The listing builds one solid part. Answer for the finished solid, in the listing's coordinates (mm). A direction names the side the tool comes from. Round coordinates to 2 decimals unless told otherwise and drop trailing zeros. Write each loop counter-clockwise with the first axis right and the second up, starting at its lowest first coordinate (ties: lowest second). Pieces come first, ordered by that corner, then holes. Notation, with made-up numbers: (39, -26) - (43, -26) arc R32 ccw to (43, 0) - close; hole circle Ø5 at (16, 10). An arc over 180 degrees is marked (long way). Return JSON: item names as keys, results as strings. Group by question number.
(1) Section C-C, the plane x = 261.5 is taken. Write down the section's boundary in (y, z), then the cut area to 3 significant figures.
(2) Determine the mould class of faces 1 (the flat face through (131, 21, 99)), 2 (the flat face through (0, 20, 50)) for opening direction X: +X half, -X half, draft (parallel to the pull), parting line (faces both ways), or undercut.
(3) Section B-B, the plane z = 53 is taken. Write down the section's boundary in (x, y).
(4) Which of the six approach directions +Z, -Z, +X, -X, +Y, -Y give full straight-line access (tool end or side, diameter ignored) to faces 3 (the flat face through (131, 40.8, 54)), 4 (the flat face through (271, 15, 94.5)), 5 (the flat face through (131, 20, 0))?
(5) Find the intervals of material crossed by line 1 along X through (y, z) = (30, 1); line 2 along Z through (x, y) = (148, 9); line 3 along Y through (x, z) = (158.5, 55), in increasing order. Write a range as [from, to].
(6) Section A-A, the plane y = 13 is taken. Write down the section's boundary in (x, z).
(7) Each of these flat-tipped pins is pushed along its axis until it touches: pin 1 (12 mm diameter, centred on x = 224, y = 20, fed in from -Z); pin 2 (0.5 mm diameter, centred on x = 265.5, z = -21, fed in from -Y); pin 3 (6 mm diameter, centred on y = 9, z = -5.5, fed in from +X). Where does it stop, or does it pass through?
Autodesk Inventor part; units mm, degrees
ref_plane "YZ Plane" through (0, 0, 0) normal (1, 0, 0) x (0, 1, 0)
ref_plane "XZ Plane" through (0, 0, 0) normal (0, 1, 0) x (-1, 0, 0)
ref_plane "XY Plane" through (0, 0, 0) normal (0, 0, 1) x (1, 0, 0)
sketch "Sketch1" plane through (0, 0, 0) normal (1, 0, 0) x (0, 1, 0)
  line L0 (0, 0) -> (40.8, 0)
  line L1 (40.8, 0) -> (40.8, 99)
  line L2 (40.8, 99) -> (0, 99)
  line L3 (0, 99) -> (0, 0)
  dimension "d0" = 40.8
  dimension "d1" = 99
extrude "Extrusion1" add sketch "Sketch1" along normal blind 265
sketch "Sketch2" plane through (265, 0, 0) normal (1, 0, 0) x (0, 0, -1)
  line L0 (0, 40.8) -> (-99, 40.8)
  line L1 (-94.5, 40.8) -> (-94.5, -1.5)
  line L2 (-94.5, -1.5) -> (-93.5, -1.5)
  line L3 (-93.5, -1.5) -> (-93.5, 1.8)
  line L4 (-93.5, 1.8) -> (14.5, 1.8)
  line L5 (14.5, 1.8) -> (18.5, 5.8)
  line L6 (18.5, 5.8) -> (26, 5.8)
  line L7 (26, 5.8) -> (26, 16.3)
  line L8 (26, 16.3) -> (18.5, 16.3)
  line L9 (18.5, 16.3) -> (14.5, 21.3)
  line L10 (14.5, 21.3) -> (18.5, 26.3)
  line L11 (18.5, 26.3) -> (26, 26.3)
  line L12 (26, 26.3) -> (26, 36.8)
  line L13 (26, 36.8) -> (18.5, 36.8)
  line L14 (18.5, 36.8) -> (14.5, 40.8)
  line L15 (14.5, 40.8) -> (0, 40.8)
  line L16 (0, 0) -> (0, 40.8)
  line L17 (0, 40.8) -> (-94.5, 40.8)
  line L18 (-99, 40.8) -> (-99, 0)
  line L19 (-99, 0) -> (0, 0)
  line L20 (14.5, 21.3) -> (14.5, 40.8) construction
  dimension "d4" = 4.5
  dimension "d5" = 1
  dimension "d6" = 1.5
  dimension "d7" = 135
  dimension "d8" = 135
  dimension "d9" = 10.5
  dimension "d10" = 4
  dimension "d11" = 7.5
  dimension "d13" = 10
  dimension "d14" = 108
extrude "Extrusion2" add sketch "Sketch2" along normal blind 1 contours L16 L4 L3 L19 L1 L0 | L15 L14 L13 L12 L11 L10 L9 L8 L7 L6 L5 L4 L16 | L19 L3 L2 L1
sketch "Sketch3" plane through (265, -1.5, 94.5) normal (0, 0, 1) x (1, 0, 0)
  line L0 (1, 42.3) -> (1, 0)
  line L1 (1, 0) -> (12.5, 0)
  line L2 (12.5, 0) -> (12.5, 8.05)
  line L3 (12.5, 8.05) -> (9.5, 8.05)
  line L4 (9.5, 8.05) -> (9.5, 11.05)
  line L5 (9.5, 11.05) -> (12.5, 11.05)
  line L6 (12.5, 11.05) -> (12.5, 28.55)
  line L7 (12.5, 28.55) -> (9.5, 28.55)
  line L8 (9.5, 28.55) -> (9.5, 31.55)
  line L9 (9.5, 31.55) -> (12.5, 31.55)
  line L10 (12.5, 31.55) -> (12.5, 39.7)
  line L11 (12.5, 39.7) -> (1, 39.7)
  line L12 (1, 39.7) -> (1, 0)
  line L13 (0, 42.3) -> (0, 1.5)
  line L14 (0, 42.3) -> (1, 42.3)
  point P0 (-265, 1.5)
  point P1 (9.5, 30.05)
  point P2 (9.5, 9.55)
  dimension "d17" = 11.5
  dimension "d18" = 12.25
  dimension "d19" = 20.5
  dimension "d20" = 3
  dimension "d21" = 3
  dimension "d22" = 3
  dimension "d23" = 2.6
extrude "Extrusion3" add sketch "Sketch3" against normal blind 1
properties part number "Vega56dummy"
Working result:
{
 "1": {"outline": "(0, 0) - (40.8, 0) - (40.8, 99) - (0, 99) - close", "area": "4,040 mm^2"},
 "2": {"face 1": "draft", "face 2": "-X half"},
 "3": {"outline": "(0, 0) - (265, 0) - (265, 1.8) - (266, 1.8) - (266, 40.8) - (0, 40.8) - close"},
 "4": {"face 3": "+Z, -Z, +X, -X, +Y", "face 4": "+Z, +X, +Y, -Y", "face 5": "-Z, -X, +Y, -Y"},
 "5": {"line 1": "x = [0, 266]", "line 2": "z = [0, 99]", "line 3": "y = [0, 40.8]"},
 "6": {"outline": "(0, 0) - (265, 0) - (265, -26) - (266, -26) - (266, 93.5) - (277.5, 93.5) - (277.5, 94.5) - (265, 94.5) - (265, 99) - (0, 99) - close"},
 "7": {"pin 1": "stops at z = 0", "pin 2": "stops at y = 5.8", "pin 3": "stops at x = 266"}
}
